Read the model definition and answer for the solid it produces. Units are mm, in the model's axes. A direction names the side the tool comes from. Coordinates: 2 decimals unless noted, no trailing zeros. Order: outer loops, then holes, each group sorted by start corner. A loop starts at its lowest first (then second) coordinate and runs counter-clockwise, first axis right, second up. Notation, with made-up numbers: (-31.5, 72) -> (-17.5, 72) arc R8 cw to (-17.5, 80) -> close; hole circle Ø3 at (-25.5, 88). An arc over 180 degrees is marked (long way). Answer in a Markdown table with one row per item.
from build123d import *

# Parameters (mm, degrees)
SKETCH7_R                = 7
BOSS_EXTRUDE1_DEPTH      = 46
CUT_EXTRUDE1_START       = -46
CUT_EXTRUDE1_OUTLINE_R   = 7
CUT_EXTRUDE1_DEPTH       = 42
M3_CLEARANCE_HOLE1_D     = 3.2
M3_CLEARANCE_HOLE1_DEPTH = 5
M3_CLEARANCE_HOLE1_TIP   = 0.96137699
M3_TAPPED_HOLE1_D        = 2.5
M3_TAPPED_HOLE1_DEPTH    = 7.5
M3_TAPPED_HOLE1_TIP      = 0.751075774
FILLET1_R                = 5


# Read off the part's stored shape, not the designer's step: Cut-Extrude1
with BuildPart() as part:
    # Sketch7 → Boss-Extrude1 (new body)
    with BuildSketch(Plane(origin=(0, 0, 0), x_dir=(0, 0, -1), z_dir=(1, 0, 0))):
        with BuildLine():
            Line((-7.5, 27.902912484), (-7.5, 30.902912484))
            ThreePointArc((-7.5, 30.902912484), (-16.218584434, 27.353199428), (-23.515946886, 21.40654671))
            ThreePointArc((-23.515946886, 21.40654671), (-26.429411238, 19.642162968), (-29.833839376, 19.747962631))
            ThreePointArc((-29.833839376, 19.747962631), (-35.912951138, 17.155172414), (-34.109592252, 10.797023497))
            ThreePointArc((-34.109592252, 10.797023497), (-31.887887506, 8.215289092), (-31.429483161, 4.840205393))
            ThreePointArc((-31.429483161, 4.840205393), (-31.8, 0), (-31.429483161, -4.840205393))
            ThreePointArc((-31.429483161, -4.840205393), (-31.887887506, -8.215289092), (-34.109592252, -10.797023497))
            ThreePointArc((-34.109592252, -10.797023497), (-35.912951138, -17.155172414), (-29.833839376, -19.747962631))
            ThreePointArc((-29.833839376, -19.747962631), (-26.429411238, -19.642162968), (-23.515946886, -21.40654671))
            ThreePointArc((-23.515946886, -21.40654671), (0, -31.8), (23.515946886, -21.40654671))
            ThreePointArc((23.515946886, -21.40654671), (26.429411238, -19.642162968), (29.833839376, -19.747962631))
            ThreePointArc((29.833839376, -19.747962631), (35.912951138, -17.155172414), (34.109592252, -10.797023497))
            ThreePointArc((34.109592252, -10.797023497), (31.887887506, -8.215289092), (31.429483161, -4.840205393))
            ThreePointArc((31.429483161, -4.840205393), (31.8, 0), (31.429483161, 4.840205393))
            ThreePointArc((31.429483161, 4.840205393), (31.887887506, 8.215289092), (34.109592252, 10.797023497))
            ThreePointArc((34.109592252, 10.797023497), (35.912951138, 17.155172414), (29.833839376, 19.747962631))
            ThreePointArc((29.833839376, 19.747962631), (26.429411238, 19.642162968), (23.515946886, 21.40654671))
            ThreePointArc((23.515946886, 21.40654671), (16.218584434, 27.353199428), (7.5, 30.902912484))
            Line((7.5, 30.902912484), (7.5, 27.902912484))
            Line((7.5, 27.902912484), (-7.5, 27.902912484))
        make_face()
        Circle(SKETCH7_R, mode=Mode.SUBTRACT)
    extrude(amount=-BOSS_EXTRUDE1_DEPTH)

    # Cut-Extrude1 outline → Cut-Extrude1 (cut)
    with BuildSketch(Plane(origin=(0, 0, 0), x_dir=(0, 0, -1), z_dir=(1, 0, 0)).offset(CUT_EXTRUDE1_START)):
        with BuildLine():
            ThreePointArc((-22.8, 19.188538246), (-29.8, 0), (-22.8, -19.188538246))
            Line((-22.8, -19.188538246), (-22.8, -22.167543842))
            ThreePointArc((-22.8, -22.167543842), (0, -31.8), (22.8, -22.167543842))
            Line((22.8, -22.167543842), (22.8, -19.188538246))
            ThreePointArc((22.8, -19.188538246), (29.8, 0), (22.8, 19.188538246))
            Line((22.8, 19.188538246), (22.8, 22.167543842))
            ThreePointArc((22.8, 22.167543842), (15.767027822, 27.615952521), (7.5, 30.902912484))
            Line((7.5, 30.902912484), (7.5, 27.902912484))
            Line((7.5, 27.902912484), (-7.5, 27.902912484))
            Line((-7.5, 27.902912484), (-7.5, 30.902912484))
            ThreePointArc((-7.5, 30.902912484), (-15.767027822, 27.615952521), (-22.8, 22.167543842))
            Line((-22.8, 22.167543842), (-22.8, 19.188538246))
        make_face()
        Circle(CUT_EXTRUDE1_OUTLINE_R, mode=Mode.SUBTRACT)
    extrude(amount=CUT_EXTRUDE1_DEPTH, mode=Mode.SUBTRACT)

    # M3 Clearance Hole1
    with Locations(Plane(origin=(0, 0, 0), x_dir=(0, 0, -1), z_dir=(1, 0, 0))):
        with Locations((-20, 2.25), (20, 2.25), (20, -17.75), (-20, -17.75)):
            Hole(M3_CLEARANCE_HOLE1_D / 2, depth=M3_CLEARANCE_HOLE1_DEPTH)
            with Locations((0, 0, -(M3_CLEARANCE_HOLE1_DEPTH + M3_CLEARANCE_HOLE1_TIP / 2))):  # 118° drill point
                Cone(0, M3_CLEARANCE_HOLE1_D / 2, M3_CLEARANCE_HOLE1_TIP, mode=Mode.SUBTRACT)

    # M3 Tapped Hole1
    with Locations(Plane.ZY.offset(46)):
        with Locations((-31.40127386, 15), (-31.40127386, -15), (31.40127386, -15), (31.40127386, 15)):
            Hole(M3_TAPPED_HOLE1_D / 2, depth=M3_TAPPED_HOLE1_DEPTH)
            with Locations((0, 0, -(M3_TAPPED_HOLE1_DEPTH + M3_TAPPED_HOLE1_TIP / 2))):  # 118° drill point
                Cone(0, M3_TAPPED_HOLE1_D / 2, M3_TAPPED_HOLE1_TIP, mode=Mode.SUBTRACT)

    # Fillet1
    # the kernel refuses this fillet: 5 mm, written as the material it adds along each edge
    with BuildSketch(Plane(origin=(0, 27.902912484, 7.5), x_dir=(0, 0, -1), z_dir=(-1, 0, 0))) as fillet1_piece_1:
        with BuildLine():
            CenterArc((4.582575695, -5), FILLET1_R, 90, 66.421821522)
            Line((0, -3), (-0.091651514, -2.96))
            ThreePointArc((-0.091651514, -2.96), (-0.1, -1.5), (-0.1, 0))
            Line((-0.1, 0), (0, 0.1))
            Line((0, 0.1), (4.582575695, 0.1))
            Line((4.582575695, 0.1), (4.582575695, 0))
        make_face()
    extrude(amount=4)
    with BuildSketch(Plane(origin=(0, 27.902912484, -7.5), x_dir=(0, 1, 0), z_dir=(-1, 0, 0))) as fillet1_piece_2:
        with BuildLine():
            CenterArc((5, -4.582575695), FILLET1_R, 113.578178478, 66.421821522)
            Line((0, -4.582575695), (-0.1, -4.582575695))
            Line((-0.1, -4.582575695), (-0.1, 0))
            Line((-0.1, 0), (0, 0.1))
            ThreePointArc((0, 0.1), (1.5, 0.1), (2.96, 0.091651514))
            Line((2.96, 0.091651514), (3, 0))
        make_face()
    extrude(amount=4)


solid = part.part
Q1. The part is cut by section C-C (y = -17.75). Write down the section's boundary in (x, z).
Outcome:
| item | result |
|---|---|
| outline | (-46, -35.58) -> (0, -35.58) -> (0, -21.6) -> (-4, -21.6) -> (-4, -23.94) -> (-46, -23.94) -> close; (-46, 23.94) -> (-4, 23.94) -> (-4, 21.6) -> (0, 21.6) -> (0, 35.58) -> (-46, 35.58) -> close; (-4, -18.4) -> (0, -18.4) -> (0, 18.4) -> (-4, 18.4) -> close |
Q2. Consider line 1 (Z direction, x = -2, y = 2); line 2 (X direction, y = 20.5, z = -10); line 3 (Z direction, x = -36, y = 0.5). Determine where each line is inside the solid, lowest interval first.
Outcome:
| item | result |
|---|---|
| line 1 | -31.74 to -21.58, -18.42 to -6.71, 6.71 to 18.42, 21.58 to 31.74 |
| line 2 | -4 to 0 |
| line 3 | -31.8 to -29.8, 29.8 to 31.8 |
Q3. The part is cut by section D-D (z = 20). Write down the section's boundary in (x, y), then the cut area to 3 significant figures.
Outcome:
| item | result |
|---|---|
| outline | (-4, -24.72) -> (0, -24.72) -> (0, -19.35) -> (-4, -19.35) -> close; (-4, -16.15) -> (0, -16.15) -> (0, 0.65) -> (-4, 0.65) -> close; (-4, 3.85) -> (0, 3.85) -> (0, 24.72) -> (-4, 24.72) -> close |
| area | 172 mm² |
Q4. For faces 1 (the face through (-25, 21, -22.8)), 2 (the face through (-46, -5, -30)), 3 (the face through (-4, 7, 6)), determine the directions among +Z, -Z, +X, -X, +Y, -Y from which every point of the face is accessible in a straight line to the end or side of a thin tool.
Outcome:
| item | result |
|---|---|
| face 1 | -X, +Y, -Y |
| face 2 | +Z, -Z, -X, +Y, -Y |
| face 3 | -X |
Q5. For a pull along Z with two mould halves and no side action, classify faces 4 (the face through (-46, -5, 30)), 5 (the face through (-42.198, 15.055, -30.152)), 6 (the face through (-22.7, -0.1, -31.8)) as pulls with the +Z half, pulls with the -Z half, needs draft (parallel to the pull), parting line crosses it, or undercut.
Outcome:
| item | result |
|---|---|
| face 4 | needs draft |
| face 5 | undercut |
| face 6 | pulls with the -Z half |
Q6. The part is cut by section B-B (x = -17). Write down the section's boundary in (y, z).
Outcome:
| item | result |
|---|---|
| outline | (-22.17, -22.8) arc R31.8 ccw to (-21.41, -23.52) arc R6 cw to (-19.75, -29.83) arc R5 ccw to (-10.8, -34.11) arc R6 cw to (-4.84, -31.43) arc R31.8 ccw to (4.84, -31.43) arc R6 cw to (10.8, -34.11) arc R5 ccw to (19.75, -29.83) arc R6 cw to (21.41, -23.52) arc R31.8 ccw to (22.17, -22.8) -> (19.19, -22.8) arc R29.8 cw to (-19.19, -22.8) -> close; (-22.17, 22.8) -> (-19.19, 22.8) arc R29.8 cw to (19.19, 22.8) -> (22.17, 22.8) arc R31.8 ccw to (21.41, 23.52) arc R6 cw to (19.75, 29.83) arc R5 ccw to (10.8, 34.11) arc R6 cw to (4.84, 31.43) arc R31.8 ccw to (-4.84, 31.43) arc R6 cw to (-10.8, 34.11) arc R5 ccw to (-19.75, 29.83) arc R6 cw to (-21.41, 23.52) arc R31.8 ccw to start |
Q7. The part is cut by section A-A (z = 0). Write down the section's boundary in (x, y), then the cut area to 3 significant figures.
Outcome:
| item | result |
|---|---|
| outline | (-4, -31.8) -> (0, -31.8) -> (0, -7) -> (-4, -7) -> close; (-4, 7) -> (0, 7) -> (0, 27.9) -> (-4, 27.9) -> close |
| area | 183 mm² |
Q8. Given pin 1 (8 mm diameter, centred on x = -24.5, y = -9.5, fed in from -Z); pin 2 (5 mm diameter, centred on x = -24.5, y = 5, fed in from -Z); pin 3 (5 mm diameter, centred on y = -17.75, z = 20, fed in from +X); pin 4 (2 mm diameter, centred on y = 15, z = -31.4, fed in from -X), each flat-ended and moving along its own axis, determine where each tip first touches the part or whether it passes through.
Outcome:
| item | result |
|---|---|
| pin 1 | z = -36.17 |
| pin 2 | z = -31.7 |
| pin 3 | x = 0 |
| pin 4 | x = -38.35 |
